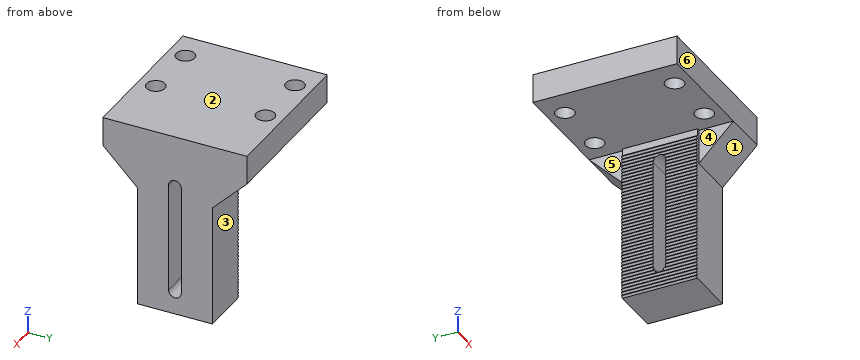
```python
from build123d import *

# Parameters (mm, degrees)
EXTRUDE_1_DEPTH          = 25
SKETCH_4_R               = 1.6
CUT_EXTRUDE_2_DEPTH      = 49.764741361
CUT_EXTRUDE_5_DEPTH      = 45.833023543
EXTRUDE_2_DEPTH          = 13
CUT_EXTRUDE_4_DEPTH      = 10
CUT_EXTRUDE_4_DEPTH_BACK = 45.833023543


with BuildPart() as part:
    # 草图1 → 凸台-拉伸1 (new body)
    with BuildSketch(Plane(origin=(0, 0, 0), x_dir=(1, 0, 0), z_dir=(0, 1, 0))):
        Polygon((0, 0), (-27, 0), (-27, 5), (-8, 5), (-8, 32), (0, 32), align=None)
    extrude(amount=EXTRUDE_1_DEPTH)

    # 草图4 → 切除-拉伸2 (cut, through all)
    with BuildSketch(Plane.XY):
        with Locations((-22, 22)):
            Circle(SKETCH_4_R)
        with Locations((-12, 22)):
            Circle(SKETCH_4_R)
        with Locations((-22, 3)):
            Circle(SKETCH_4_R)
        with Locations((-12, 3)):
            Circle(SKETCH_4_R)
    extrude(amount=-CUT_EXTRUDE_2_DEPTH, mode=Mode.SUBTRACT)

    # 草图8 → 切除-拉伸5 (cut, through all)
    with BuildSketch(Plane.ZY.offset(8)):
        Polygon((-32, 19), (-11, 19), (-5, 25), (-32, 25), align=None)
        Polygon((-11, 6), (-5, 0), (-32, 0), (-32, 6), align=None)
    extrude(amount=-CUT_EXTRUDE_5_DEPTH, mode=Mode.SUBTRACT)

    # 草图11 → 凸台-拉伸2 (add)
    with BuildSketch(Plane.XZ.offset(-6)):
        Polygon((-8, -5), (-8, -32), (-8.5, -32), (-8.8, -31.7), (-8.5, -31.4), (-8.8, -31.1), (-8.5, -30.8), (-8.8, -30.5), (-8.5, -30.2), (-8.8, -29.9), (-8.5, -29.6), (-8.8, -29.3), (-8.5, -29), (-8.8, -28.7), (-8.5, -28.4), (-8.8, -28.1), (-8.5, -27.8), (-8.8, -27.5), (-8.5, -27.2), (-8.8, -26.9), (-8.5, -26.6), (-8.8, -26.3), (-8.5, -26), (-8.8, -25.7), (-8.5, -25.4), (-8.8, -25.1), (-8.5, -24.8), (-8.8, -24.5), (-8.5, -24.2), (-8.8, -23.9), (-8.5, -23.6), (-8.8, -23.3), (-8.5, -23), (-8.8, -22.7), (-8.5, -22.4), (-8.8, -22.1), (-8.5, -21.8), (-8.8, -21.5), (-8.5, -21.2), (-8.8, -20.9), (-8.5, -20.6), (-8.8, -20.3), (-8.5, -20), (-8.8, -19.7), (-8.5, -19.4), (-8.8, -19.1), (-8.5, -18.8), (-8.8, -18.5), (-8.5, -18.2), (-8.8, -17.9), (-8.5, -17.6), (-8.8, -17.3), (-8.5, -17), (-8.8, -16.7), (-8.5, -16.4), (-8.8, -16.1), (-8.5, -15.8), (-8.8, -15.5), (-8.5, -15.2), (-8.8, -14.9), (-8.5, -14.6), (-8.8, -14.3), (-8.5, -14), (-8.8, -13.7), (-8.5, -13.4), (-8.8, -13.1), (-8.5, -12.8), (-8.8, -12.5), (-8.5, -12.2), (-8.8, -11.9), (-8.5, -11.6), (-8.8, -11.3), (-8.5, -11), (-8.8, -10.7), (-8.5, -10.4), (-8.8, -10.1), (-8.5, -9.8), (-8.8, -9.5), (-8.5, -9.2), (-8.8, -8.9), (-8.5, -8.6), (-8.8, -8.3), (-8.5, -8), (-8.8, -7.7), (-8.5, -7.4), (-8.8, -7.1), (-8.5, -6.8), (-8.8, -6.5), (-8.5, -6.2), (-8.5, -5), align=None)
    extrude(amount=-EXTRUDE_2_DEPTH)

    # 草图6 → 切除-拉伸4 (cut, two sides: drawn at the far end of the back side and taken through both)
    with BuildSketch(Plane.ZY.offset(8).offset(-CUT_EXTRUDE_4_DEPTH_BACK)):
        with BuildLine():
            Line((-28, 13.6), (-9, 13.6))
            ThreePointArc((-9, 13.6), (-7.9, 12.5), (-9, 11.4))
            Line((-9, 11.4), (-28, 11.4))
            ThreePointArc((-28, 11.4), (-29.1, 12.5), (-28, 13.6))
        make_face()
    extrude(amount=CUT_EXTRUDE_4_DEPTH + CUT_EXTRUDE_4_DEPTH_BACK, mode=Mode.SUBTRACT)


solid = part.part
```
The listing builds one solid part. Answer for the finished solid, in the listing's coordinates (mm). Face numbers are marked on the shaded views. A direction names the side the tool comes from. Round coordinates to 2 decimals unless told otherwise and drop trailing zeros. Loops run counter-clockwise (first coordinate to the right, second up) from the corner with the lowest first, then second, coordinate; pieces in that order, holes last. Notation, with made-up numbers: (1.5, 8.5) - (54.5, 8.5) arc R3 cw to (54.5, 13.5) - close; hole circle Ø4 at (-37.75, 45). An arc over 180 degrees is marked (long way). Return JSON: item names as keys, results as strings. Group by question number.
1. Which of the six approach directions +Z, -Z, +X, -X, +Y, -Y give full straight-line access (tool end or side, diameter ignored) to the marked faces 4, 5 and 6?
2. The mould has two halves that part along Z. Classify the marked faces 1, 2 and 3: pulls with the +Z half, pulls with the -Z half, needs draft (parallel to the pull), parting line crosses it, or undercut.
3. Consider probe 1 along Y at (x, z) = (-22, -3.5); probe 2 along Y at (x, z) = (-6.5, -20.5); probe 3 along X at (y, z) = (21, -1.5). Determine where each line is inside the solid, lowest interval first.
4. Each of these flat-tipped pins is pushed along its axis until it touches: P1, Ø4, axis at x = -22, y = 22, coming from the -Z side; P2, Ø9.5, axis at x = -5.5, z = -18.5, coming from the +Y side; P3, Ø2.5, axis at x = -6.5, z = -18, coming from the -Y side. Where does it stop, or does it pass through?
5. The part is cut by section C-C on x = -2. Determine the outline of the cut face in (y, z).
6. The part is cut by section D-D on x = -25. Determine the outline of the cut face in (y, z).
7. The part is cut by section B-B on y = 3. Determine the outline of the cut face in (x, z).
8. The part is cut by section A-A on x = -12. Determine the outline of the cut face in (y, z).
Resolved:
{
 "1": {"face 4": "-Z, -X, -Y", "face 5": "-Z, -X, +Y", "face 6": "+Z, -Z, +X, -X, -Y"},
 "2": {"face 1": "pulls with the -Z half", "face 2": "pulls with the +Z half", "face 3": "needs draft"},
 "3": {"probe 1": "y = 0 to 1.4, 4.6 to 20.4, 23.6 to 25", "probe 2": "y = 6 to 11.4, 13.6 to 19", "probe 3": "x = -27 to -23.25, -20.75 to -13.25, -10.75 to 0"},
 "4": {"P1": "stops at z = -5", "P2": "stops at y = 19", "P3": "stops at y = 6"},
 "5": {"outline": "(0, -5) - (6, -11) - (6, -32) - (19, -32) - (19, -11) - (25, -5) - (25, 0) - (0, 0) - close; hole (11.4, -28) arc R1.1 ccw to (13.6, -28) - (13.6, -9) arc R1.1 ccw to (11.4, -9) - close"},
 "6": {"outline": "(0, -5) - (25, -5) - (25, 0) - (0, 0) - close"},
 "7": {"outline": "(-27, -5) - (-23.6, -5) - (-23.6, 0) - (-27, 0) - close; (-20.4, -5) - (-13.6, -5) - (-13.6, 0) - (-20.4, 0) - close; (-10.4, -5) - (-8, -5) - (-8, -8) - (0, -8) - (0, 0) - (-10.4, 0) - close"},
 "8": {"outline": "(0, -5) - (1.4, -5) - (1.4, 0) - (0, 0) - close; (4.6, -5) - (20.4, -5) - (20.4, 0) - (4.6, 0) - close; (23.6, -5) - (25, -5) - (25, 0) - (23.6, 0) - close"}
}
